Check sheet for the modelled part. Datum: model origin and axes. Units: mm. Face numbers are marked on the shaded views. A direction names the side the tool comes from. Give positions to 0.01 mm unless a question says otherwise; leave off trailing zeros. Write each loop counter-clockwise with the first axis right and the second up, starting at its lowest first coordinate (ties: lowest second). Pieces come first, ordered by that corner, then holes. Notation, with made-up numbers: M -13.5,-30.5 L 15.5,-30.5 A20 ccw 15.5,-8.5 Z; hole C 61.25,78.5 d5. An arc over 180 degrees is marked long. Write item = value, one per line. Start each with the question number.
1) Scan lines: L1, parallel to X at y = 22.8, z = -9; L2, parallel to X at y = 22, z = 0; L3, parallel to Z at x = -16.5, y = 22.85. Record each from-to range of solid material in increasing order.
2) Draft check along Z on the marked faces 4, 5, 6 and 7. Enter one of: pulls with the +Z half, pulls with the -Z half, needs draft (parallel to the pull), parting line crosses it, or undercut.
3) Sectioned sample at A-A, the plane x = 8. Record the cut outline in (y, z), then the cut area to 3 significant figures.
4) Sectioned sample at D-D, the plane x = -16.5. Record the cut outline in (y, z), then the cut area to 3 significant figures.
5) Set-up check for the marked faces 1, 2 and 3: record each of +Z, -Z, +X, -X, +Y, -Y from which the full face is reachable in a straight line by a thin tool's end or side.
6) Gauge pin test, flat ends, axial feed: pin 1 (0.5 mm diameter, centred on y = 1.5, z = -12, fed in from +X); pin 2 (5 mm diameter, centred on y = 13.5, z = 4, fed in from +X); pin 3 (0.6 mm diameter, centred on x = 54.5, y = 9.5, fed in from -Z). Record the tip position at first contact, or that the pin passes through.
7) Sectioned sample at B-B, the plane y = 9. Record the cut outline in (x, z).
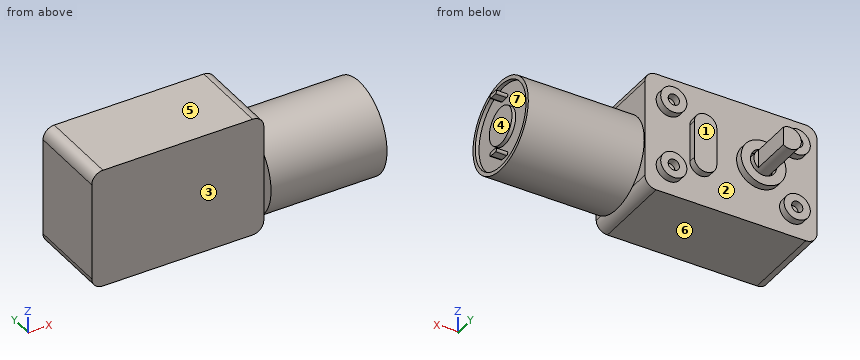
from build123d import *

# Parameters (mm, degrees)
SKETCH1_W           = 46
SKETCH1_H           = 32
BOSS_EXTRUDE1_DEPTH = 21.5
FILLET1_R           = 3
SKETCH2_R           = 3.5
SKETCH2_R_2         = 1.5
SKETCH2_R_3         = 6
BOSS_EXTRUDE2_DEPTH = 2
SKETCH3_R           = 3
BOSS_EXTRUDE3_DEPTH = 13.7
CUT_EXTRUDE1_DEPTH  = 11
SKETCH6_R           = 12.2
BOSS_EXTRUDE5_DEPTH = 31
SKETCH7_R           = 11.2
SKETCH7_R_2         = 5
CUT_EXTRUDE2_DEPTH  = 1
BOSS_EXTRUDE6_DEPTH = 3
CIRPATTERN1_COUNT   = 2


with BuildPart() as part:
    # Sketch1 → Boss-Extrude1 (new body)
    with BuildSketch(Plane(origin=(0, 0, 0), x_dir=(1, 0, 0), z_dir=(0, 1, 0))):
        Rectangle(SKETCH1_W, SKETCH1_H)
    extrude(amount=BOSS_EXTRUDE1_DEPTH)

    # Fillet1
    fillet1_edges = [part.edges().sort_by_distance(p)[0] for p in [
        (23, 10.75, 16),
        (-23, 10.75, 16),
        (-23, 10.75, -16),
        (23, 10.75, -16),
    ]]
    fillet(fillet1_edges, radius=FILLET1_R)

    # Sketch2 → Boss-Extrude2 (add)
    with BuildSketch(Plane(origin=(0, 21.5, 0), x_dir=(1, 0, 0), z_dir=(0, 1, 0))):
        with Locations((-16.5, 9)):
            Circle(SKETCH2_R)
        with Locations((-16.5, 9)):
            Circle(SKETCH2_R_2, mode=Mode.SUBTRACT)
        with Locations((16.5, 9)):
            Circle(SKETCH2_R)
        with Locations((16.5, 9)):
            Circle(SKETCH2_R_2, mode=Mode.SUBTRACT)
        with Locations((16.5, -9)):
            Circle(SKETCH2_R)
        with Locations((16.5, -9)):
            Circle(SKETCH2_R_2, mode=Mode.SUBTRACT)
        with Locations((-16.5, -9)):
            Circle(SKETCH2_R)
        with Locations((-16.5, -9)):
            Circle(SKETCH2_R_2, mode=Mode.SUBTRACT)
        with Locations((-7.5, 0)):
            Circle(SKETCH2_R_3)
        with Locations((-7.5, 0)):
            Circle(SKETCH2_R, mode=Mode.SUBTRACT)
        with BuildLine():
            Line((11, 5), (11, -5))
            ThreePointArc((11, -5), (8, -8), (5, -5))
            Line((5, -5), (5, 5))
            ThreePointArc((5, 5), (8, 8), (11, 5))
        make_face()
    extrude(amount=BOSS_EXTRUDE2_DEPTH)

    # Sketch3 → Boss-Extrude3 (add)
    with BuildSketch(Plane(origin=(0, 21.5, 0), x_dir=(1, 0, 0), z_dir=(0, 1, 0))):
        with Locations((-7.5, 0)):
            Circle(SKETCH3_R)
    extrude(amount=BOSS_EXTRUDE3_DEPTH)

    # Sketch4 → Cut-Extrude1 (cut)
    with BuildSketch(Plane(origin=(0, 35.2, 0), x_dir=(1, 0, 0), z_dir=(0, 1, 0))):
        Polygon((-5.7, 80.583575735), (-5.7, 2.4), (-5.7, -2.4), (-5.7, -80.583575735), (150.66715147, -80.583575735), (150.66715147, 80.583575735), align=None)
    extrude(amount=-CUT_EXTRUDE1_DEPTH, mode=Mode.SUBTRACT)

    # Sketch6 → Boss-Extrude5 (add)
    with BuildSketch(Plane(origin=(23, 0, 0), x_dir=(0, 0, -1), z_dir=(1, 0, 0))):
        with Locations((3, 9)):
            Circle(SKETCH6_R)
    extrude(amount=BOSS_EXTRUDE5_DEPTH)

    # Sketch7 → Cut-Extrude2 (cut)
    with BuildSketch(Plane(origin=(54, 0, 0), x_dir=(0, 0, -1), z_dir=(1, 0, 0))):
        with Locations((3, 9)):
            Circle(SKETCH7_R)
        with Locations((3, 9)):
            Circle(SKETCH7_R_2, mode=Mode.SUBTRACT)
    extrude(amount=-CUT_EXTRUDE2_DEPTH, mode=Mode.SUBTRACT)

    # Sketch8 → Boss-Extrude6 (add)
    with BuildSketch(Plane(origin=(53, 0, 0), x_dir=(0, 0, -1), z_dir=(1, 0, 0))):
        with BuildLine():
            Line((-5.5, 8), (-5.5, 10))
            ThreePointArc((-5.5, 10), (-5, 10.5), (-4.5, 10))
            Line((-4.5, 10), (-4.5, 8))
            ThreePointArc((-4.5, 8), (-5, 7.5), (-5.5, 8))
        make_face()
    boss_extrude6 = extrude(amount=BOSS_EXTRUDE6_DEPTH)

    # CirPattern1: Boss-Extrude6 ×2 about axis
    cirpattern1_axis = Axis((0, 9, -3), (1, 0, 0))
    for i in range(1, CIRPATTERN1_COUNT):
        add(boss_extrude6.rotate(cirpattern1_axis, i * 360 / CIRPATTERN1_COUNT))


solid = part.part
Data:
q1.L1 = -20 to -18, -15 to -13, 13 to 15, 18 to 20
q1.L2 = -13.5 to -11, -10.5 to -4.5, -4 to -1.5, 5 to 11
q1.L3 = -12.5 to -10.5, -7.5 to -5.5, 5.5 to 7.5, 10.5 to 12.5
q2.face_4 = undercut
q2.face_5 = pulls with the +Z half
q2.face_6 = pulls with the -Z half
q2.face_7 = undercut
q3.outline = M 0,-16 L 21.5,-16 L 21.5,-8 L 23.5,-8 L 23.5,8 L 21.5,8 L 21.5,16 L 0,16 Z
q3.area = 720 mm2
q4.outline = M 0,-16 L 21.5,-16 L 21.5,-12.5 L 23.5,-12.5 L 23.5,-10.5 L 21.5,-10.5 L 21.5,-7.5 L 23.5,-7.5 L 23.5,-5.5 L 21.5,-5.5 L 21.5,5.5 L 23.5,5.5 L 23.5,7.5 L 21.5,7.5 L 21.5,10.5 L 23.5,10.5 L 23.5,12.5 L 21.5,12.5 L 21.5,16 L 0,16 Z
q4.area = 704 mm2
q5.face_1 = +Z, -Z, +X, +Y
q5.face_2 = +Y
q5.face_3 = +Z, -Z, -X, -Y
q6.pin_1 = 54
q6.pin_2 = 53
q6.pin_3 = -11.5
q7.outline = M -23,-13 A3 ccw -20,-16 L 20,-16 A3 ccw 23,-13 L 23,-15.2 L 54,-15.2 L 54,-14.2 L 53,-14.2 L 53,-11.5 L 56,-11.5 L 56,-10.5 L 53,-10.5 L 53,-8 L 54,-8 L 54,2 L 53,2 L 53,4.5 L 56,4.5 L 56,5.5 L 53,5.5 L 53,8.2 L 54,8.2 L 54,9.2 L 23,9.2 L 23,13 A3 ccw 20,16 L -20,16 A3 ccw -23,13 Z
